Study the drawing (mm; zero at the part's minimum x, y, z) and answer. A direction names the side the tool comes from. Round coordinates to 2 decimals unless told otherwise and drop trailing zeros. Write each loop counter-clockwise with the first axis right and the second up, starting at its lowest first coordinate (ties: lowest second). Pieces come first, ordered by that corner, then holes. Notation, with made-up numbers: (75.5, -22) -> (87.5, -22) arc R29 ccw to (87.5, -2) -> close; hole circle Ø11 at (17.25, 6). An arc over 180 degrees is marked (long way). Return JSON: item names as keys, results as strings.
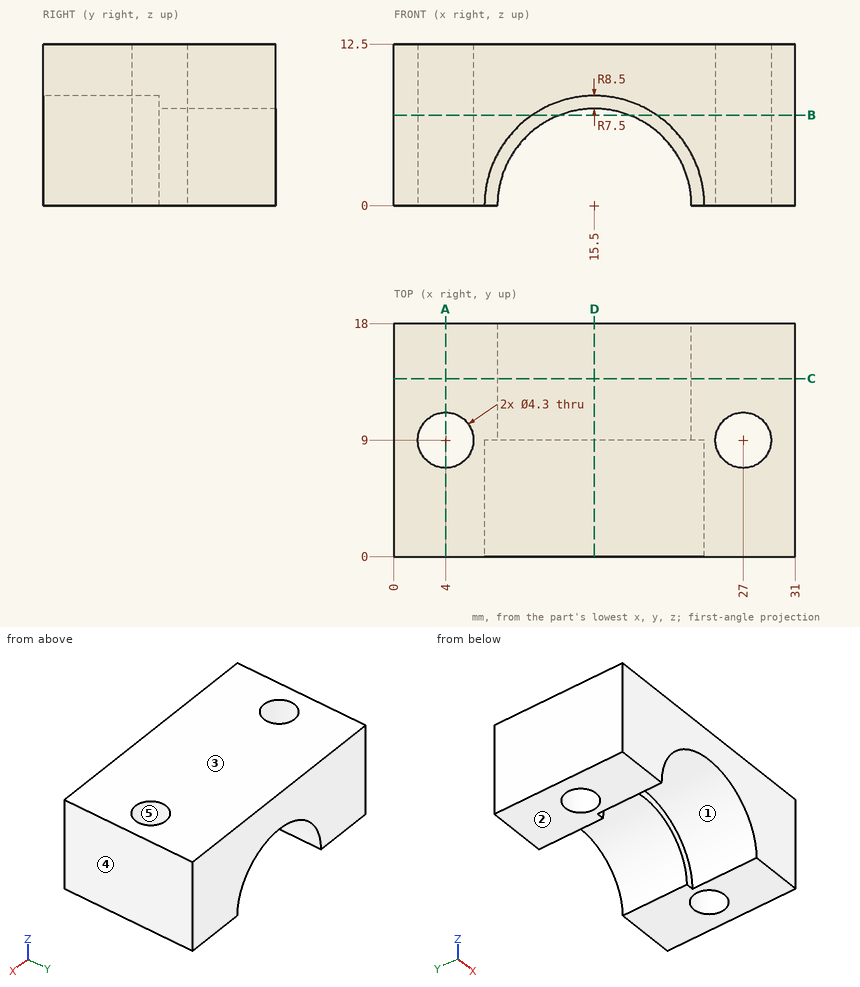
Item 1: Section C-C (y = 13.75) is taken. Give the vertices of the cut face in (x, z).
Worked answers:
{"outline": "(0, 0) -> (8, 0) arc R7.5 cw to (23, 0) -> (31, 0) -> (31, 12.5) -> (0, 12.5) -> close"}
Item 2: Section D-D (x = 15.5) is taken. Give the vertices of the cut face in (y, z).
Worked answers:
{"outline": "(0, 8.5) -> (9, 8.5) -> (9, 7.5) -> (18, 7.5) -> (18, 12.5) -> (0, 12.5) -> close"}
Item 3: Section A-A (x = 4) is taken. Give the vertices of the cut face in (y, z), then the cut area to 3 significant figures.
Worked answers:
{"outline": "(0, 0) -> (6.85, 0) -> (6.85, 12.5) -> (0, 12.5) -> close; (11.15, 0) -> (18, 0) -> (18, 12.5) -> (11.15, 12.5) -> close", "area": "171 mm2"}
Item 4: Straight lines are drawn through the part: L1, parallel to X at y = 9, z = 8.5; L2, parallel to Y at x = 27, z = 8.5; L3, parallel to X at y = 10.25, z = 11.5. For each, find the intervals that lie inside material, in ascending order. Write a range as [from, to].
Worked answers:
{"L1": "x = [0, 1.85], [6.15, 24.85], [29.15, 31]", "L2": "y = [0, 6.85], [11.15, 18]", "L3": "x = [0, 2.25], [5.75, 25.25], [28.75, 31]"}
Item 5: Flat-ended cylindrical pins translate along their axes: pin 1 (6 mm diameter, centred on x = 21.5, z = 1.5, fed in from -Y); pin 2 (5 mm diameter, centred on x = 12.5, y = 7, fed in from -Z); pin 3 (4 mm diameter, centred on x = 13.5, z = 5.5, fed in from -Y). Find the tip coordinate at first contact, or state that the pin passes through.
Worked answers:
{"pin 1": "stops at y = 0", "pin 2": "stops at z = 6", "pin 3": "stops at y = 9"}
Item 6: Section B-B (z = 7) is taken. Give the vertices of the cut face in (x, y), then the cut area to 3 significant figures.
Worked answers:
{"outline": "(0, 0) -> (10.68, 0) -> (10.68, 9) -> (12.81, 9) -> (12.81, 18) -> (0, 18) -> close; (18.19, 9) -> (20.32, 9) -> (20.32, 0) -> (31, 0) -> (31, 18) -> (18.19, 18) -> close; hole circle Ø4.3 at (4, 9); hole circle Ø4.3 at (27, 9)", "area": "394 mm2"}
Item 7: For a pull along X with two mould halves and no side action, classify the marked faces 3, 4 and 5 as released by +X, released by -X, zero draft, split by the parting line, or undercut.
Worked answers:
{"face 3": "zero draft", "face 4": "released by +X", "face 5": "undercut"}
Item 8: A tool of negligible diameter and unlimited length cuts with its end or side. For the marked faces 1 and 2, from which of +Z, -Z, +X, -X, +Y, -Y can it reach the whole face along a straight path? Write none if from no direction.
Worked answers:
{"face 1": "-Z, -Y", "face 2": "-Z, +X, -X, +Y, -Y"}
